```python
from build123d import *

# Parameters (mm, degrees)
F0_W     = 25
F0_H     = 81
F0_W_2   = 20
F0_H_2   = 75
F1_DEPTH = 8
F2_W     = 8
F2_H     = 2
F3_DEPTH = 8
F5_R     = 6
F6_W     = 22.5
F6_H     = 20
F7_DEPTH = 1.5
F8_R     = 0.75
F9_DEPTH = 100


with BuildPart() as f1:
    # F0 (on Top) → F1 (new body)
    with BuildSketch(Plane.XY):
        Rectangle(F0_W, F0_H)
        Rectangle(F0_W_2, F0_H_2, mode=Mode.SUBTRACT)
    extrude(amount=F1_DEPTH)

    # F2 (on face) → F3 (join)
    with BuildSketch(Plane.XY.offset(8)):
        with Locations((-6, 33)):
            Rectangle(F2_W, F2_H)
        with Locations((6, 33)):
            Rectangle(F2_W, F2_H)
    extrude(amount=-F3_DEPTH)

    # F5
    f5_edges = [f1.edges().sort_by_distance(p)[0] for p in [
        (-12.5, 40.5, 4),
        (12.5, 40.5, 4),
        (12.5, -40.5, 4),
        (-12.5, -40.5, 4),
    ]]
    fillet(f5_edges, radius=F5_R)

    # F6 (on face) → F7 (join)
    with BuildSketch(Plane.XY.offset(8)):
        with Locations((-1.25, 0)):
            Rectangle(F6_W, F6_H)
    extrude(amount=-F7_DEPTH)

    # F8 (on face) → F9 (cut)
    with BuildSketch(Plane.XZ.offset(40.5)):
        with Locations((0, 4)):
            Circle(F8_R)
    extrude(amount=-F9_DEPTH, mode=Mode.SUBTRACT)


solid = f1.part
```
Model file for the job. Use its own axes, mm. A direction names the side the tool comes from. Round coordinates to 2 decimals unless told otherwise and drop trailing zeros. Write each loop counter-clockwise with the first axis right and the second up, starting at its lowest first coordinate (ties: lowest second). Pieces come first, ordered by that corner, then holes. Notation, with made-up numbers: (-37.5, 72.25) -> (20.5, 72.25) arc R8 ccw to (20.5, 85.25) -> close; hole circle Ø9 at (-9, -30). An arc over 180 degrees is marked (long way). Answer as CSV lines item,"result".
1. Slice it at B-B, the plane z = 4. List the corners of the cut face in (x, y), plus the area to 3 significant figures.
Resolved:
outline,"(-12.5, -34.5) arc R6 ccw to (-6.5, -40.5) -> (-0.75, -40.5) -> (-0.75, -37.5) -> (-10, -37.5) -> (-10, 32) -> (-2, 32) -> (-2, 34) -> (-10, 34) -> (-10, 37.5) -> (-0.75, 37.5) -> (-0.75, 40.5) -> (-6.5, 40.5) arc R6 ccw to (-12.5, 34.5) -> close; (0.75, -40.5) -> (6.5, -40.5) arc R6 ccw to (12.5, -34.5) -> (12.5, 34.5) arc R6 ccw to (6.5, 40.5) -> (0.75, 40.5) -> (0.75, 37.5) -> (10, 37.5) -> (10, 34) -> (2, 34) -> (2, 32) -> (10, 32) -> (10, -37.5) -> (0.75, -37.5) -> close"
area,"517 mm²"
2. Slice it at A-A, the plane x = 0. List the corners of the cut face in (y, z), plus the area to 3 significant figures.
Resolved:
outline,"(-40.5, 0) -> (-37.5, 0) -> (-37.5, 3.25) -> (-40.5, 3.25) -> close; (-40.5, 4.75) -> (-37.5, 4.75) -> (-37.5, 8) -> (-40.5, 8) -> close; (-10, 6.5) -> (10, 6.5) -> (10, 8) -> (-10, 8) -> close; (37.5, 0) -> (40.5, 0) -> (40.5, 3.25) -> (37.5, 3.25) -> close; (37.5, 4.75) -> (40.5, 4.75) -> (40.5, 8) -> (37.5, 8) -> close"
area,"69.0 mm²"
3. Drill centre lines: line 1 (Y direction, x = -6, z = 6); line 2 (Z direction, x = 0, y = -38.2); line 3 (X direction, y = -30, z = 7.5). Where is each one in solid material? Low to high.
Resolved:
line 1,"-40.5 to -37.5, 32 to 34, 37.5 to 40.5"
line 2,"0 to 3.25, 4.75 to 8"
line 3,"-12.5 to -10, 10 to 12.5"
4. Tool access for faces 1 (the face through (-12.5, 0, 4)), 2 (the face through (6, 32, 4)): list every direction of +Z, -Z, +X, -X, +Y, -Y with a clear straight run to the whole face (end or side of a thin tool).
Resolved:
face 1,"+Z, -Z, -X, +Y, -Y"
face 2,"+Z, -Z"
5. Pin check, flat tips, straight feed: pin 1 Ø6 at (x, y) = (-4, 3) entering from -Z; pin 2 Ø2 at (x, z) = (9, 2.5) entering from +Y. Stop position of each tip, or through.
Resolved:
pin 1,"z = 6.5"
pin 2,"y = 40.31"
6. Mould opens along Z. For faces 3 (the face through (-0.163, 38.979, 3.268)), 4 (the face through (0, 0, 6.5)), 5 (the face through (-10, -3, 4)) say: +Z half, -Z half, draft (parallel to the pull), parting line (faces both ways), or undercut.
Resolved:
face 3,"undercut"
face 4,"-Z half"
face 5,"draft"
7. Slice it at C-C, the plane y = 13. List the corners of the cut face in (x, z).
Resolved:
outline,"(-12.5, 0) -> (-10, 0) -> (-10, 8) -> (-12.5, 8) -> close; (10, 0) -> (12.5, 0) -> (12.5, 8) -> (10, 8) -> close"
8. Slice it at D-D, the plane x = 7.5. List the corners of the cut face in (y, z), plus the area to 3 significant figures.
Resolved:
outline,"(-40.42, 0) -> (-37.5, 0) -> (-37.5, 8) -> (-40.42, 8) -> close; (-10, 6.5) -> (10, 6.5) -> (10, 8) -> (-10, 8) -> close; (32, 0) -> (34, 0) -> (34, 8) -> (32, 8) -> close; (37.5, 0) -> (40.42, 0) -> (40.42, 8) -> (37.5, 8) -> close"
area,"92.7 mm²"
